Design review of the part built by this model. Coordinates are the model's own, in mm. A direction names the side the tool comes from. Give positions to 0.01 mm unless a question says otherwise; leave off trailing zeros. Loops run counter-clockwise (first coordinate to the right, second up) from the corner with the lowest first, then second, coordinate; pieces in that order, holes last. Notation, with made-up numbers: (30, 73.25) - (73, 73.25) arc R20 ccw to (73, 93.25) - close; hole circle Ø5 at (47.25, 14). An arc over 180 degrees is marked (long way). Write each question's results on one line, items separated by ' | '.
```python
from build123d import *

# Parameters (mm, degrees)
F0_W        = 25
F0_H        = 12.5
F0_R        = 2.5
F1_DEPTH    = 5
F3_DEPTH    = 1
F4_DEPTH    = 3
F5_T4_DEPTH = 38.037750089


# Not quite as in the source:
# - a fillet or chamfer that OpenCascade refuses, or shapes differently, is made with other operations: its cross-section is extruded or revolved along the edge and cut away or added


with BuildPart() as f1:
    # F0 (on Front) → F1 (new body)
    with BuildSketch(Plane.XZ):
        with Locations((-6.15, 0)):
            Rectangle(F0_W, F0_H)
        Circle(F0_R, mode=Mode.SUBTRACT)
    extrude(amount=F1_DEPTH)

    # F2 (on face) → F3 (join)
    with BuildSketch(Plane(origin=(-18.65, 0, 0), x_dir=(0, -1, 0), z_dir=(-1, 0, 0))):
        Polygon((0, 6.25), (0, -6.25), (5, -6.25), (5, 6.25), (2.5, 6.25), align=None)
        Polygon((-12.8557521937, 21.5708888624), (0, 6.25), (2.5, 6.25), (-12.3952659434, 21.5708888624), align=None)
        Polygon((2.5, 6.25), (5, 6.25), (17.8557521937, 21.5708888624), (15.3557521937, 21.5708888624), align=None)
    extrude(amount=-F3_DEPTH)

    # F2 (on face) → F4 (join)
    with BuildSketch(Plane(origin=(-18.65, 0, 0), x_dir=(0, -1, 0), z_dir=(-1, 0, 0))):
        Polygon((0, 6.25), (0, -6.25), (5, -6.25), (5, 6.25), (2.5, 6.25), align=None)
        Polygon((-12.8557521937, 21.5708888624), (0, 6.25), (2.5, 6.25), (-12.3952659434, 21.5708888624), align=None)
        Polygon((-35.0204582804, 42.2711459978), (0, 6.25), (-12.8557521937, 21.5708888624), (-12.3952659434, 21.5708888624), (-35.0532565039, 44.8763173483), align=None)
        Polygon((2.5, 6.25), (5, 6.25), (17.8557521937, 21.5708888624), (15.3557521937, 21.5708888624), align=None)
        Polygon((-12.3952659434, 21.5708888624), (2.5, 6.25), (15.3557521937, 21.5708888624), align=None)
        Polygon((15.3557521937, 21.5708888624), (17.8557521937, 21.5708888624), (35.2253303214, 42.2711459978), (34.9467307814, 44.9185079767), align=None)
    extrude(amount=F4_DEPTH)

    # F5: chamfer of 2 on 1 edges, made by hand


with BuildPart() as f5_tool2:
    # F5_s3 → F5_t4 (new body)
    with BuildSketch(Plane.XZ.offset(20.4991181697)):
        Polygon((-18.65, 19.5708888624), (-20.65, 21.5708888624), (-18.65, 21.5708888624), align=None)
    extrude(amount=-F5_T4_DEPTH)

    split(bisect_by=Plane(origin=(0, -4.4089680227, 4.2864844086), x_dir=(1, 0, 0), z_dir=(0, -0.7169959169, 0.6970773667)), keep=Keep.TOP)

    split(bisect_by=Plane(origin=(0, 1.6104640061, 1.3513397535), x_dir=(1, 0, 0), z_dir=(0, 0.7660444431, 0.6427876097)), keep=Keep.TOP)


with BuildPart() as f1_1:
    add(f1.part)

    # F5_t1: cut F5_tool2
    add(f5_tool2.part, mode=Mode.SUBTRACT)


solid = f1_1.part
```
Item 1: We need section B-B on x = 0. Give the boundary of the cut face in (y, z), then the cut area to 3 significant figures.
Output values:
outline: (-5, -6.25) - (0, -6.25) - (0, -2.5) - (-5, -2.5) - close; (-5, 2.5) - (0, 2.5) - (0, 6.25) - (-5, 6.25) - close | area: 37.5 mm²
Item 2: Clearance check with flat-ended pins moving along their axes: P1, Ø7.5, axis at y = -8, z = 16, coming from the +X side; P2, Ø8, axis at x = 0, z = 0, coming from the -Y side; P3, Ø10, axis at x = -1, z = -2, coming from the +Y side; P4, Ø10, axis at x = 2.5, y = -6.5, coming from the -Z side. State where each tip first meets the part, or that it passes through.
Output values:
P1: stops at x = -17.65 | P2: stops at y = -5 | P3: stops at y = 0 | P4: stops at z = -6.25
Item 3: Draft analysis for pull direction X (two halves, no side actions). For faces 4 (the face through (6.35, -2, 0)), 5 (the face through (-21.65, -3, 19)), 6 (the face through (-6, -2, 6.25)), 7 (the face through (-0.54, -2.46, -2.44)), state which applies: +X half, -X half, draft (parallel to the pull), parting line (faces both ways), or undercut.
Output values:
face 4: +X half | face 5: -X half | face 6: draft | face 7: undercut
Item 4: We need section D-D on y = 7. Give the boundary of the cut face in (x, z), then the cut area to 3 significant figures.
Output values:
outline: (-21.65, 13.45) - (-18.65, 13.45) - (-18.65, 14.59) - (-17.65, 14.59) - (-17.65, 16.02) - (-18.65, 16.02) - (-18.65, 19.57) - (-20.65, 21.57) - (-21.65, 21.57) - close | area: 23.8 mm²
Item 5: Wall thickness on probe 1 along Z at (x, y) = (0, -2.8); probe 2 along Y at (x, z) = (-10.25, 4.5): over which ranges is each line inside the solid? List them lowest first.
Output values:
probe 1: z = -6.25 to -2.5, 2.5 to 6.25 | probe 2: y = -5 to 0
Item 6: We need section C-C on y = -4. Give the boundary of the cut face in (x, z), then the cut area to 3 significant figures.
Output values:
outline: (-21.65, -6.25) - (6.35, -6.25) - (6.35, 6.25) - (-17.65, 6.25) - (-17.65, 8.04) - (-18.65, 8.04) - (-18.65, 19.57) - (-20.65, 21.57) - (-21.65, 21.57) - close; hole circle Ø5 at (0, 0) | area: 376 mm²
Item 7: We need section A-A on z = 0. Give the boundary of the cut face in (x, y).
Output values:
outline: (-21.65, -5) - (-2.5, -5) - (-2.5, 0) - (-21.65, 0) - close; (2.5, -5) - (6.35, -5) - (6.35, 0) - (2.5, 0) - close
Item 8: Tool access review of faces 1 (the face through (-17.65, 4, 12)), 2 (the face through (-18.65, -1, 16)), 3 (the face through (-7, -5, 0)): name each direction out of +Z, -Z, +X, -X, +Y, -Y from which nothing blocks a thin tool from reaching the whole face with its end or side.
Output values:
face 1: +Z, +X, +Y, -Y | face 2: +Z, +X | face 3: -Z, +X, -X, -Y
